Geometry: final body of the model. Coordinates: model frame, mm. A direction names the side the tool comes from. Round coordinates to 2 decimals unless told otherwise and drop trailing zeros. Write each loop counter-clockwise with the first axis right and the second up, starting at its lowest first coordinate (ties: lowest second). Pieces come first, ordered by that corner, then holes. Notation, with made-up numbers: M 61.25,59 L 75.25,59 A16 cw 75.25,66 Z; hole C -6,50 d5. An arc over 180 degrees is marked long. Answer as CSV lines item,"result". Start each with the question number.
Q1. Section query B-B on y = 27. Output: boundary loops of the cut face in (x, z).
Q2. Ray query, probe 1 along Z at (x, y) = (0, 39.5); probe 2 along Y at (x, z) = (-43.5, 32.5); probe 3 along Z at (x, y) = (0, 58). Return the intervals inside material, ascending.
Q3. Reachability of faces 1 (the cylindrical face through (-26.76, 95.07, 51.46)), 2 (the cylindrical face through (-47.69, 14.79, -15.02)), 3 (the cylindrical face through (6.9, 57.54, -52.55)) from +Z, -Z, +X, -X, +Y, -Y: full face, straight path, thin tool, end or side. Return the list, or none.
Q4. First-contact query: pin 1 (5 mm diameter, centred on x = 41, z = -24.5, fed in from +Y); pin 2 (8 mm diameter, centred on y = 25.5, z = 41, fed in from -X); pin 3 (1 mm diameter, centred on x = -44, z = 17.5, fed in from -Y). Flat tips, straight axial feed; report the tip coordinate or a pass-through.
Q5. Mould query, pull axis X, two halves, no side actions, for faces 4 (the flat face through (-26, 65, 47)), 5 (the flat face through (22, 30, -37.3)), 6 (the cylindrical face through (6.9, 77.54, -52.55)). Classes: pulls with the +X half, pulls with the -X half, needs draft (parallel to the pull), parting line crosses it, or undercut.
Q6. Section query A-A on y = 57.5. Output: boundary loops of the cut face in (x, z), and give its area (3 significant figures).
```python
from build123d import *


with BuildPart() as part:
    # Sketch1 → Revolve1 (revolve)
    with BuildSketch(Plane.XY, mode=Mode.PRIVATE) as revolve1_sk:
        with BuildLine():
            Line((50, 0), (58, 0))
            Line((58, 0), (58, 55))
            Line((58, 55), (53, 55))
            Line((53, 55), (53, 60))
            Line((53, 60), (58, 60))
            Line((58, 60), (58, 65))
            Line((58, 65), (53, 65))
            Line((53, 65), (53, 70))
            Line((53, 70), (58, 70))
            Line((58, 70), (58, 75))
            Line((58, 75), (53, 75))
            Line((53, 75), (53, 80))
            Line((53, 80), (58, 80))
            Line((58, 80), (58, 85))
            Line((58, 85), (53, 85))
            Line((53, 85), (53, 90))
            Line((53, 90), (58, 90))
            Line((58, 90), (58, 100))
            ThreePointArc((58, 100), (29.445044376, 107.630676018), (0, 110.200125156))
            Line((0, 110.200125156), (0, 103.200125156))
            ThreePointArc((0, 103.200125156), (21.692969078, 101.750164131), (43, 97.426077213))
            Line((43, 97.426077213), (43, 30))
            Line((43, 30), (50, 30))
            Line((50, 30), (50, 0))
        make_face()
    revolve(revolve1_sk.sketch.rotate(Axis((0, 0, 0), (0, -1, 0)), 180), axis=Axis((0, 0, 0), (0, -1, 0)))


solid = part.part
```
Entries:
1,outline,"C 0,0 d116; hole C 0,0 d100"
2,probe 1,"z = -58 to -43, 43 to 58"
2,probe 2,"y = 0 to 55, 60 to 65, 70 to 75, 80 to 85, 90 to 101.29"
2,probe 3,"z = -53 to -43, 43 to 53"
3,face 1,"+Y, -Y"
3,face 2,"-Y"
3,face 3,"none"
4,pin 1,"stops at y = 104.06"
4,pin 2,"stops at x = -44.67"
4,pin 3,"stops at y = 30"
5,face 4,"needs draft"
5,face 5,"undercut"
5,face 6,"parting line crosses it"
6,outline,"C 0,0 d106; hole C 0,0 d86"
6,area,"3,020 mm^2"
